For this review, use the dimensioned drawing (mm, ordinates from the lowest corner) and the shaded views. Give positions to 0.01 mm unless a question says otherwise; leave off trailing zeros. Loops run counter-clockwise (first coordinate to the right, second up) from the corner with the lowest first, then second, coordinate; pieces in that order, holes last. Notation, with made-up numbers: M 67,80.25 L 98,80.25 A20 ccw 98,119.25 Z; hole C 25.25,-2 d7. An arc over 180 degrees is marked long. Use CSV: the item, a comma, the result in double quotes. Start each with the question number.
1. Take a section at D-D, the plane x = 12. Write out the cut boundary in (y, z).
2. Take a section at A-A, the plane y = 5. Write out the cut boundary in (x, z) (1 decimal), and give its area (3 significant figures).
3. To check wall thickness, follow line 1 (Z direction, x = 100.5, y = 5) (1 decimal); line 2 (Z direction, x = 76.5, y = 3.75) (1 decimal); line 3 (X direction, y = 0.5, z = 65) (1 decimal). State the ranges of each line that lie inside material, in increasing order. Write a range as [from, to].
4. Take a section at C-C, the plane x = 59.5. Write out the cut boundary in (y, z).
5. Take a section at B-B, the plane z = 77.5. Write out the cut boundary in (x, y), and give its area (3 significant figures).
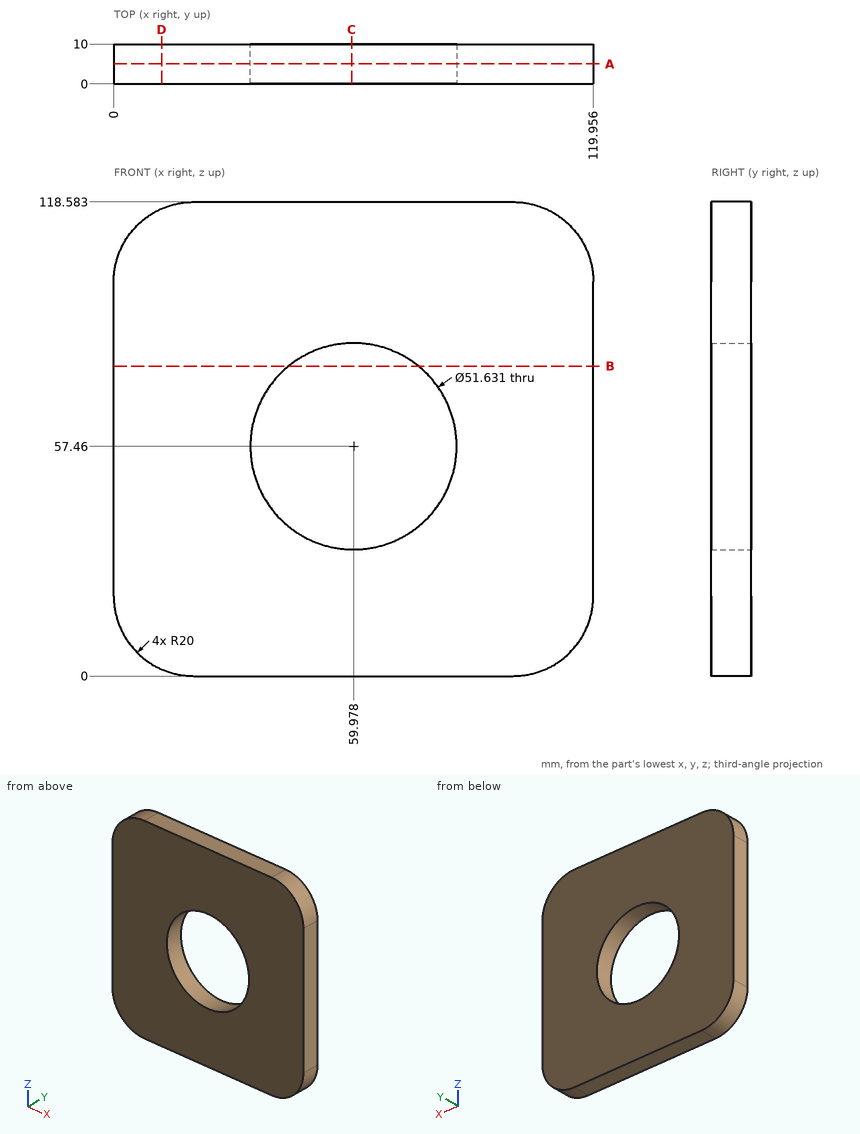
Result set:
1,outline,"M 0,1.67 L 10,1.67 L 10,116.91 L 0,116.91 Z"
2,outline,"M 0,20 A20 ccw 20,0 L 100,0 A20 ccw 120,20 L 120,98.6 A20 ccw 100,118.6 L 20,118.6 A20 ccw 0,98.6 Z; hole C 60,57.5 d51.6"
2,area,"11,800 mm2"
3,line 1,"[0, 118.6]"
3,line 2,"[0, 37.6], [77.3, 118.6]"
3,line 3,"[0, 35.3], [84.7, 120]"
4,outline,"M 0,0 L 10,0 L 10,31.65 L 0,31.65 Z; M 0,83.27 L 10,83.27 L 10,118.58 L 0,118.58 Z"
5,outline,"M 0,0 L 43.7,0 L 43.7,10 L 0,10 Z; M 76.25,0 L 119.96,0 L 119.96,10 L 76.25,10 Z"
5,area,"874 mm2"
